```python
from build123d import *

# Parameters (mm, degrees)
CROQUIS1_W              = 1206.08
CROQUIS1_H              = 80
CROQUIS1_R              = 4.7625
CROQUIS1_R_2            = 4.765
SALIENTE_EXTRUIR1_DEPTH = 10
CROQUIS2_W              = 1206.08
CROQUIS2_H              = 10
SALIENTE_EXTRUIR2_DEPTH = 70
CROQUIS3_R              = 4.765
CORTAR_EXTRUIR1_DEPTH   = 1211.755535358
CORTAR_EXTRUIR2_DEPTH   = 15
CORTAR_EXTRUIR3_DEPTH   = 15


with BuildPart() as part:
    # Croquis1 → Saliente-Extruir1 (new body)
    with BuildSketch(Plane.XY):
        with Locations((603.04, 40)):
            Rectangle(CROQUIS1_W, CROQUIS1_H)
        with Locations((30, 40)):
            Circle(CROQUIS1_R, mode=Mode.SUBTRACT)
        with Locations((1176.08, 40)):
            Circle(CROQUIS1_R_2, mode=Mode.SUBTRACT)
    extrude(amount=SALIENTE_EXTRUIR1_DEPTH)

    # Croquis2 → Saliente-Extruir2 (add)
    with BuildSketch(Plane.XY.offset(10)):
        with Locations((603.04, 75)):
            Rectangle(CROQUIS2_W, CROQUIS2_H)
    extrude(amount=SALIENTE_EXTRUIR2_DEPTH)

    # Croquis3 → Cortar-Extruir1 (cut, through all)
    with BuildSketch(Plane.XZ.offset(-70)):
        with Locations((1182.956834807, 45)):
            Circle(CROQUIS3_R)
        with Locations((43.661184758, 45)):
            Circle(CROQUIS3_R)
    extrude(amount=-CORTAR_EXTRUIR1_DEPTH, mode=Mode.SUBTRACT)

    # Croquis4 → Cortar-Extruir2 (cut)
    with BuildSketch(Plane(origin=(1206.08, 0, 0), x_dir=(0, 0, -1), z_dir=(1, 0, 0))):
        Polygon((-10, 0), (0, 0), (0, 80), (-80, 80), (-80, 70), (-10, 70), align=None)
    extrude(amount=-CORTAR_EXTRUIR2_DEPTH, mode=Mode.SUBTRACT)

    # Croquis5 → Cortar-Extruir3 (cut)
    with BuildSketch(Plane.ZY):
        Polygon((0, 80), (0, 0), (10, 0), (10, 70), (80, 70), (80, 80), align=None)
    extrude(amount=-CORTAR_EXTRUIR3_DEPTH, mode=Mode.SUBTRACT)


solid = part.part
```
The listing builds one solid part. Answer for the finished solid, in the listing's coordinates (mm). A direction names the side the tool comes from. Give positions to 0.01 mm unless a question says otherwise; leave off trailing zeros. Loops run counter-clockwise (first coordinate to the right, second up) from the corner with the lowest first, then second, coordinate; pieces in that order, holes last. Notation, with made-up numbers: (28, 54.25) - (63, 54.25) arc R8 ccw to (63, 65.25) - close; hole circle Ø9 at (-36, 3). An arc over 180 degrees is marked (long way). Return JSON: item names as keys, results as strings. Group by question number.
1. Find section A-A (x = 962). Write down the section's boundary in (y, z).
2. Given pin 1 Ø11 at (x, z) = (43.66, 45) entering from -Y; pin 2 Ø21 at (x, y) = (665.5, 25.5) entering from +Z, each flat-ended and moving along its own axis, determine where each tip first touches the part or whether it passes through.
3. Which of the six approach directions +Z, -Z, +X, -X, +Y, -Y give full straight-line access (tool end or side, diameter ignored) to faces 1 (the flat face through (595, 35, 10)), 2 (the flat face through (595, 80, 39))?
4. Straight lines are drawn through the part: line 1 (Y direction, x = 1176, z = 2); line 2 (Z direction, x = 158, y = 38.5); line 3 (Y direction, x = 545, z = 21). For each, find the intervals that lie inside material, in ascending order. Write a range as [from, to].
Verdict:
{
 "1": {"outline": "(0, 0) - (80, 0) - (80, 80) - (70, 80) - (70, 10) - (0, 10) - close"},
 "2": {"pin 1": "stops at y = 70", "pin 2": "stops at z = 10"},
 "3": {"face 1": "+Z, +X, -X, -Y", "face 2": "+Z, -Z, +X, -X, +Y"},
 "4": {"line 1": "y = [0, 35.24], [44.76, 80]", "line 2": "z = [0, 10]", "line 3": "y = [70, 80]"}
}
